Design review of the part shown in the three views and the two pictorial views. Dimensions are in mm from the part's minimum x, y and z. A direction names the side the tool comes from. Coordinates: 2 decimals unless noted, no trailing zeros. Loops run counter-clockwise (first coordinate to the right, second up) from the corner with the lowest first, then second, coordinate; pieces in that order, holes last. Notation, with made-up numbers: M 88,-19 L 99,-19 A22 cw 99,12 Z; hole C 15,-24.5 d4. An arc over 180 degrees is marked long. Put each result on its own line as item: value. Start each with the question number.
(1) Take a section at C-C, the plane y = 7.25. Give the boundary of the cut face in (x, z).
(2) Clearance check with flat-ended pins moving along their axes: pin 1 (1.5 mm diameter, centred on x = 47, z = 30, fed in from -Y); pin 2 (17.5 mm diameter, centred on x = 20, z = 22, fed in from +Y). State where each tip first meets the part, or that it passes through.
(3) Take a section at D-D, the plane z = 29. Give the boundary of the cut face in (x, y).
(4) The part is to be moulded in two halves that separate along X. For the marked faces 3, 4 and 5, say which applies: +X half, -X half, draft (parallel to the pull), parting line (faces both ways), or undercut.
(5) Take a section at A-A, the plane z = 35. Give the boundary of the cut face in (x, y).
(6) Take a section at B-B, the plane x = 40. Give the boundary of the cut face in (y, z), then the cut area to 4 significant figures.
(7) For the marked faces 1 and 2, list the 3-axis set-ups (+Z, -Z, +X, -X, +Y, -Y) from which the entire face can be reached by the end or side of a thin tool; tool diameter is ignored.
(8) For probe 1 along Z at (x, y) = (10.5, 4.25); probe 2 along X at (y, z) = (6.25, 37); probe 3 along Y at (x, z) = (53.5, 31.5), list the stretches that pass through material, from the lowest coordinate up. Write a range as [from, to].
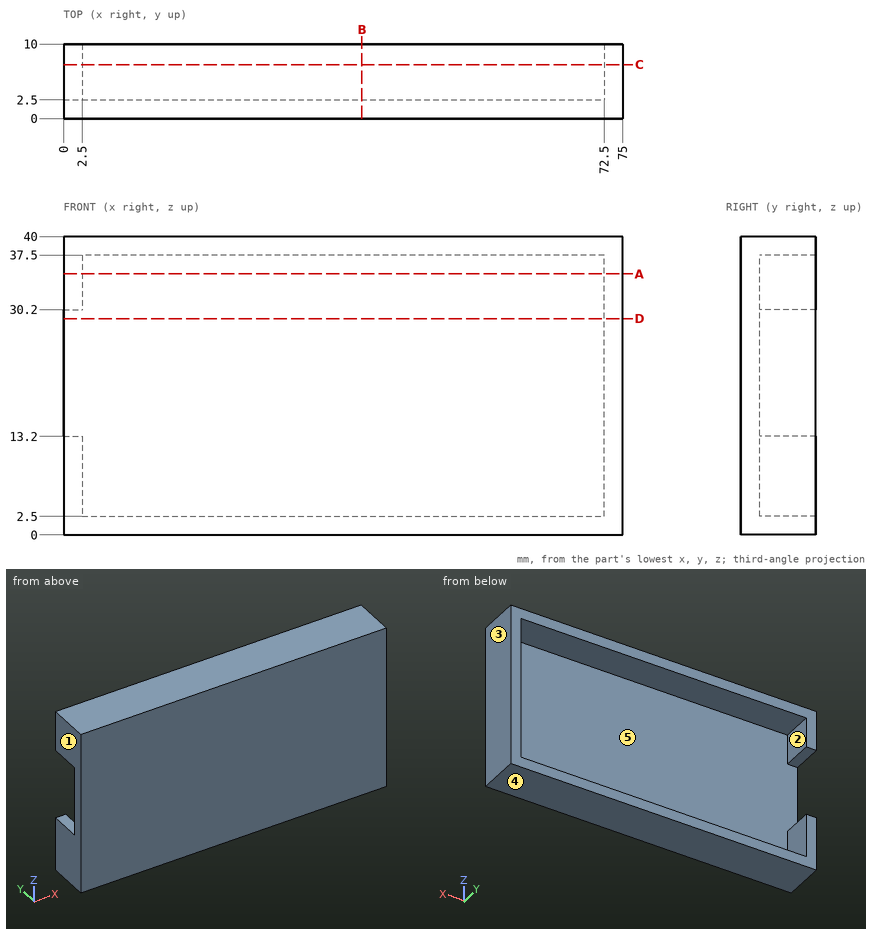
Computed values:
1. outline: M 0,0 L 75,0 L 75,40 L 0,40 L 0,30.2 L 2.5,30.2 L 2.5,37.5 L 72.5,37.5 L 72.5,2.5 L 2.5,2.5 L 2.5,13.2 L 0,13.2 Z
2. pin 1: stops at y = 0
2. pin 2: stops at y = 2.5
3. outline: M 0,0 L 75,0 L 75,10 L 72.5,10 L 72.5,2.5 L 0,2.5 Z
4. face 3: +X half
4. face 4: draft
4. face 5: undercut
5. outline: M 0,0 L 75,0 L 75,10 L 72.5,10 L 72.5,2.5 L 2.5,2.5 L 2.5,10 L 0,10 Z
6. outline: M 0,0 L 10,0 L 10,2.5 L 2.5,2.5 L 2.5,37.5 L 10,37.5 L 10,40 L 0,40 Z
6. area: 137.5 mm^2
7. face 1: +Z, -Z, -X, +Y, -Y
7. face 2: +Y
8. probe 1: z = [0, 2.5], [37.5, 40]
8. probe 2: x = [0, 2.5], [72.5, 75]
8. probe 3: y = [0, 2.5]
